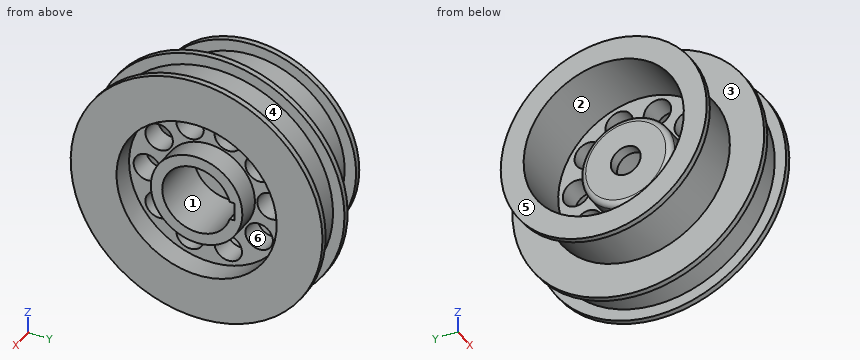
```python
from build123d import *

# Parameters (mm, degrees)
BOSS_EXTRUDE1_DEPTH      = 15
BOSS_EXTRUDE1_DEPTH_BACK = 15
SKETCH1_R                = 20
SKETCH2_R                = 20
SKETCH2_R_2              = 6.5
BOSS_EXTRUDE2_DEPTH      = 5
BOSS_EXTRUDE3_DEPTH      = 5
BOSS_EXTRUDE3_DEPTH_BACK = 5
SKETCH3_R                = 40
SKETCH3_R_2              = 6
SKETCH3_R_3              = 17.5
FILLET1_R                = 2.5


with BuildPart() as part:
    # Sketch1 → Boss-Extrude1 (new, two sides: drawn at the far end of the back side and taken through both)
    with BuildSketch(Plane(origin=(0, 0, 0), x_dir=(0, 0, -1), z_dir=(1, 0, 0)).offset(-BOSS_EXTRUDE1_DEPTH_BACK)):
        Circle(SKETCH1_R)
        with BuildLine():
            Line((-4, 14.456832295), (-4, 16.5))
            Line((-4, 16.5), (4, 16.5))
            Line((4, 16.5), (4, 14.456832295))
            ThreePointArc((4, 14.456832295), (0, -15), (-4, 14.456832295))
        make_face(mode=Mode.SUBTRACT)
    extrude(amount=BOSS_EXTRUDE1_DEPTH + BOSS_EXTRUDE1_DEPTH_BACK)

    # Sketch2 → Boss-Extrude2 (add)
    with BuildSketch(Plane.ZY.offset(15)):
        with Locations(Location((0, 0, 0), (0, 0, 180))):
            Circle(SKETCH2_R)
        Circle(SKETCH2_R_2, mode=Mode.SUBTRACT)
    extrude(amount=-BOSS_EXTRUDE2_DEPTH)

    # Sketch3 → Boss-Extrude3 (add, two sides: drawn at the far end of the back side and taken through both)
    with BuildSketch(Plane(origin=(0, 0, 0), x_dir=(0, 0, -1), z_dir=(1, 0, 0)).offset(-BOSS_EXTRUDE3_DEPTH_BACK)):
        Circle(SKETCH3_R)
        with Locations((0, 27)):
            Circle(SKETCH3_R_2, mode=Mode.SUBTRACT)
        Circle(SKETCH3_R_3, mode=Mode.SUBTRACT)
        with Locations((15.870201812, 21.843458848)):
            Circle(SKETCH3_R_2, mode=Mode.SUBTRACT)
        with Locations((25.67852594, 8.343458848)):
            Circle(SKETCH3_R_2, mode=Mode.SUBTRACT)
        with Locations((25.67852594, -8.343458848)):
            Circle(SKETCH3_R_2, mode=Mode.SUBTRACT)
        with Locations((15.870201812, -21.843458848)):
            Circle(SKETCH3_R_2, mode=Mode.SUBTRACT)
        with Locations((0, -27)):
            Circle(SKETCH3_R_2, mode=Mode.SUBTRACT)
        with Locations((-15.870201812, -21.843458848)):
            Circle(SKETCH3_R_2, mode=Mode.SUBTRACT)
        with Locations((-25.67852594, -8.343458848)):
            Circle(SKETCH3_R_2, mode=Mode.SUBTRACT)
        with Locations((-25.67852594, 8.343458848)):
            Circle(SKETCH3_R_2, mode=Mode.SUBTRACT)
        with Locations((-15.870201812, 21.843458848)):
            Circle(SKETCH3_R_2, mode=Mode.SUBTRACT)
    extrude(amount=BOSS_EXTRUDE3_DEPTH + BOSS_EXTRUDE3_DEPTH_BACK)

    # Sketch5 → Revolve1 (revolve)
    with BuildSketch(Plane.XY, mode=Mode.PRIVATE) as revolve1_sk:
        Polygon((-32.5, 35), (-32.5, 45), (-30, 45), (-30, 40), (-5, 40), (-5, 55), (-2.5, 55), (-2.5, 50), (12.5, 50), (12.5, 55), (15, 55), (15, 35), align=None)
    revolve(revolve1_sk.sketch.rotate(Axis((0, 0, 0), (1, 0, 0)), 90), axis=Axis((0, 0, 0), (1, 0, 0)))

    # Fillet1
    fillet1_edges = [part.edges().sort_by_distance(p)[0] for p in [
        (-15, 0, 20),
    ]]
    fillet(fillet1_edges, radius=FILLET1_R)


solid = part.part
```
For this review, take the finished solid that the model builds, in its own axes (mm). Face numbers are marked on the shaded views. A direction names the side the tool comes from. Round coordinates to 2 decimals unless told otherwise and drop trailing zeros. Order: outer loops, then holes, each group sorted by start corner. A loop starts at its lowest first (then second) coordinate and runs counter-clockwise, first axis right, second up. Notation, with made-up numbers: (25, 59) -> (35, 59) arc R23 cw to (35, 90) -> close; hole circle Ø5 at (30, 78.25). An arc over 180 degrees is marked (long way). Use a Markdown table: item, result.
Item 1: For line 1 along Y through (x, z) = (0, 0); line 2 along X through (y, z) = (42, 4); line 3 along Y through (x, z) = (7.5, 0), list the stretches that pass through material, from the lowest coordinate up. Write a range as [from, to].
Resolved:
| item | result |
|---|---|
| line 1 | y = [-50, -33], [-21, -15], [16.5, 21], [33, 50] |
| line 2 | x = [-32.5, -30], [-5, 15] |
| line 3 | y = [-50, -35], [-20, -15], [16.5, 20], [35, 50] |
Item 2: Draft analysis for pull direction Z (two halves, no side actions). For the marked faces 4, 5 and 6, state which applies: +Z half, -Z half, draft (parallel to the pull), parting line (faces both ways), or undercut.
Resolved:
| item | result |
|---|---|
| face 4 | parting line |
| face 5 | draft |
| face 6 | undercut |
Item 3: Take a section at B-B (z = 47.5). State the section outline as (x, y) points.
Resolved:
| item | result |
|---|---|
| outline | (-5, -27.73) -> (-2.5, -27.73) -> (-2.5, -15.61) -> (12.5, -15.61) -> (12.5, -27.73) -> (15, -27.73) -> (15, 27.73) -> (12.5, 27.73) -> (12.5, 15.61) -> (-2.5, 15.61) -> (-2.5, 27.73) -> (-5, 27.73) -> close |
Item 4: Take a section at A-A (x = 8.5). State the section outline as (y, z) points.
Resolved:
| item | result |
|---|---|
| outline | circle Ø100 at (0, 0); circle Ø40 at (0, 0); hole circle Ø70 at (0, 0); hole (14.46, -4) -> (16.5, -4) -> (16.5, 4) -> (14.46, 4) arc R15 ccw (long way) to start |
Item 5: Machinability: for the marked faces 1, 2 and 3, which of the approach directions +Z, -Z, +X, -X, +Y, -Y give a long, thin tool a straight path to every point of the face, cutting with its end or side? Answer none if there is none.
Resolved:
| item | result |
|---|---|
| face 1 | +X |
| face 2 | -X |
| face 3 | none |
Item 6: For pin 1 (10.5 mm diameter, centred on y = -7.5, z = 7, fed in from -X); pin 2 (5 mm diameter, centred on x = 4, z = 11, fed in from +Y); pin 3 (1.5 mm diameter, centred on x = 7.5, z = -2, fed in from +Y), all flat-tipped, find the tip position at first contact; note any pin that passes through.
Resolved:
| item | result |
|---|---|
| pin 1 | stops at x = -15 |
| pin 2 | stops at y = 49.27 |
| pin 3 | stops at y = 49.98 |
Item 7: Take a section at C-C (x = 2). State how many separate pieces and enclosed holes the cut face has, plus the area to 3 significant figures.
Resolved:
| item | result |
|---|---|
| separate pieces | 1 |
| enclosed holes | 11 |
| area | 6,000 mm² |
